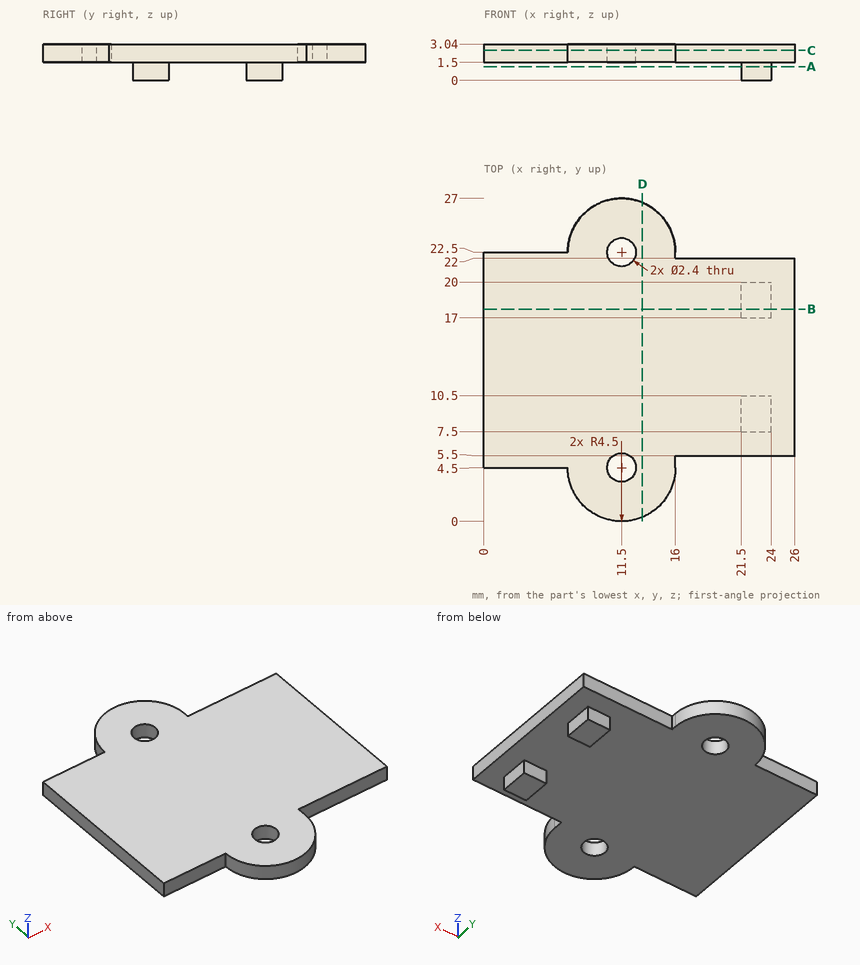
Source: three-view drawing plus pictorial views. Frame: mm from the lowest corner of the part. Coordinates: 2 decimals unless noted, no trailing zeros. Loops run counter-clockwise (first coordinate to the right, second up) from the corner with the lowest first, then second, coordinate; pieces in that order, holes last. Notation, with made-up numbers: (-2.5, -18.5) - (52.5, -18.5) arc R23 cw to (52.5, 15.5) - close; hole circle Ø6 at (40, 51.5). An arc over 180 degrees is marked (long way). Answer in a Markdown table with one row per item. Add a question column.
Item 1: Section query D-D on x = 13.25. Return the cut outline in (y, z), then the cut area to 3 significant figures.
Item 2: Section query C-C on z = 2.5. Return the cut outline in (x, y), then the cut area to 3 significant figures.
Item 3: Section query A-A on z = 1.15. Return the cut outline in (x, y), then the cut area to 3 significant figures.
Item 4: Contact query for flat-ended pins moving along their axis: P1, Ø0.5, axis at y = 9, z = 0.5, coming from the +X side; P2, Ø0.8, axis at x = 23, z = 1, coming from the -Y side; P3, Ø0.8, axis at x = 22.5, z = 2.5, coming from the +Y side; P4, Ø1.9, axis at x = 11.5, y = 4.5, coming from the +Z side. Output: stop coordinate, or through.
Item 5: Section query B-B on y = 17.75. Return the cut outline in (x, z), then the cut area to 3 significant figures.
Item 6: Line query: line 1 along Y through (x, z) = (11.75, 2.25); line 2 along Z through (x, y) = (9, 9.5); line 3 along Y through (x, z) = (5.25, 2.8). Output: solid intervals per line, ascending. Write a range as [from, to].
Recorded:
| question | item | result |
|---|---|---|
| 1 | outline | (0.35, 1.5) - (26.65, 1.5) - (26.65, 3.04) - (0.35, 3.04) - close |
| 1 | area | 40.5 mm^2 |
| 2 | outline | (0, 4.5) - (7, 4.5) arc R4.5 ccw to (16, 4.5) - (16, 5.5) - (26, 5.5) - (26, 22) - (16, 22) - (16, 22.5) arc R4.5 ccw to (7, 22.5) - (0, 22.5) - close; hole circle Ø2.4 at (11.5, 4.5); hole circle Ø2.4 at (11.5, 22.5) |
| 2 | area | 508 mm^2 |
| 3 | outline | (21.5, 7.5) - (24, 7.5) - (24, 10.5) - (21.5, 10.5) - close; (21.5, 17) - (24, 17) - (24, 20) - (21.5, 20) - close |
| 3 | area | 15.0 mm^2 |
| 4 | P1 | x = 24 |
| 4 | P2 | y = 7.5 |
| 4 | P3 | y = 22 |
| 4 | P4 | through |
| 5 | outline | (0, 1.5) - (21.5, 1.5) - (21.5, 0) - (24, 0) - (24, 1.5) - (26, 1.5) - (26, 3.04) - (0, 3.04) - close |
| 5 | area | 43.8 mm^2 |
| 6 | line 1 | [0.01, 3.33], [5.67, 21.33], [23.67, 26.99] |
| 6 | line 2 | [1.5, 3.04] |
| 6 | line 3 | [4.5, 22.5] |
